Could you check a few things on this drawing? It's one solid part, dimensions in mm from its lowest x, y, z. A direction names the side the tool comes from. Give positions to 0.01 mm unless a question says otherwise; leave off trailing zeros. Order: outer loops, then holes, each group sorted by start corner. A loop starts at its lowest first (then second) coordinate and runs counter-clockwise, first axis right, second up. Notation, with made-up numbers: (40.5, -19.75) -> (92.5, -19.75) arc R7 ccw to (92.5, -10.75) -> close; hole circle Ø4 at (-27, -18). An arc over 180 degrees is marked (long way). Answer as a JSON object with one key per item and string values.
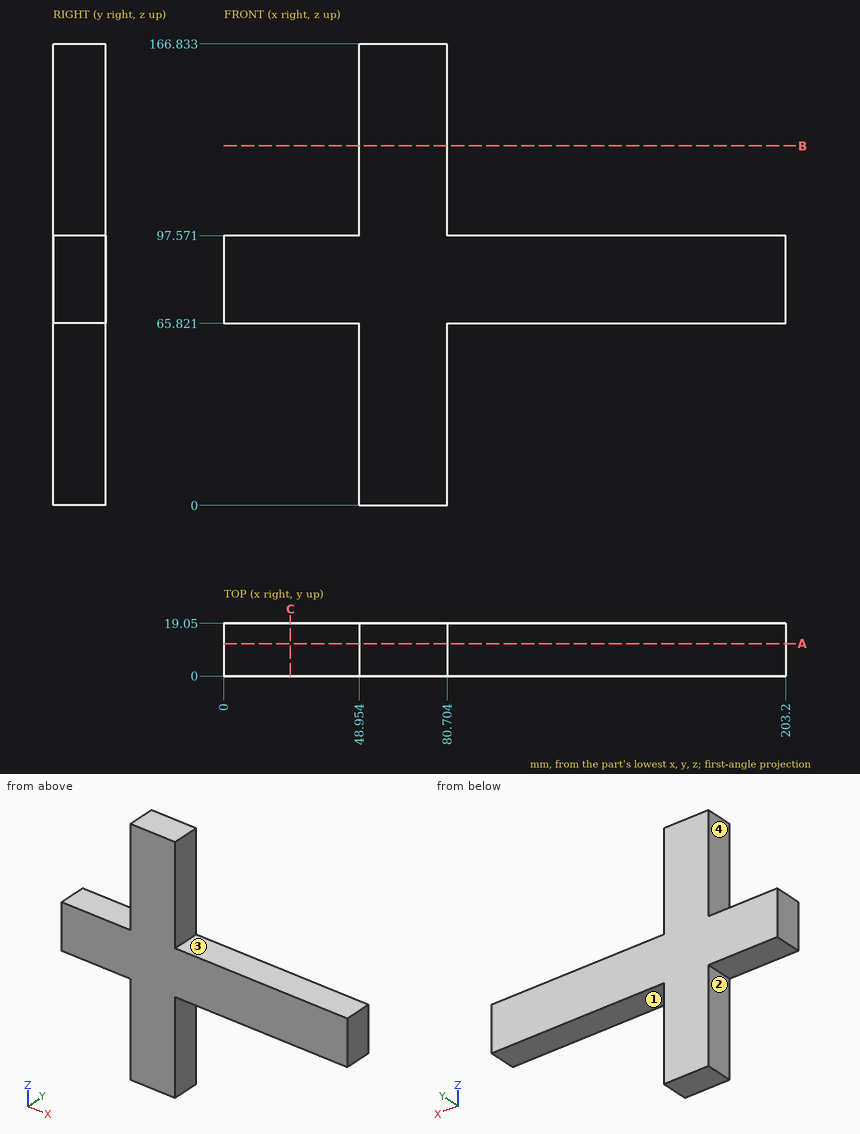
1. Please list where these lines run through material, in increasing order: L1, parallel to Z at x = 43, y = 10.25; L2, parallel to X at y = 15.75, z = 132.5.
Worked answers:
{"L1": "65.82 to 97.57", "L2": "48.95 to 80.7"}
2. If we section it at C-C on x = 24: Please give me the cut outline in (y, z).
Worked answers:
{"outline": "(0, 65.82) -> (19.05, 65.82) -> (19.05, 97.57) -> (0, 97.57) -> close"}
3. For the marked faces 1, 2, 3 and 4, which set-ups out of +Z, -Z, +X, -X, +Y, -Y let a thin tool reach every point of the face, with its end or its side?
Worked answers:
{"face 1": "-Z, +X, +Y, -Y", "face 2": "-Z, -X, +Y, -Y", "face 3": "+Z, +X, +Y, -Y", "face 4": "+Z, -X, +Y, -Y"}
4. Will these pins go through, and if not, where does the flat tip stop? pin 1 Ø1 at (y, z) = (13, 53.5) entering from +X; pin 2 Ø3 at (x, y) = (127.5, 15) entering from -Z; pin 3 Ø1 at (x, y) = (132, 13) entering from +Z; pin 4 Ø12 at (x, z) = (128.5, 108) entering from +Y.
Worked answers:
{"pin 1": "x = 80.7", "pin 2": "z = 65.82", "pin 3": "z = 97.57", "pin 4": "through"}
5. If we section it at B-B on z = 130: Please give me the cut outline in (x, y), then the cut area to 3 significant figures.
Worked answers:
{"outline": "(48.95, 0) -> (80.7, 0) -> (80.7, 19.05) -> (48.95, 19.05) -> close", "area": "605 mm²"}
6. If we section it at A-A on y = 11.75: Please give me the cut outline in (x, z).
Worked answers:
{"outline": "(0, 65.82) -> (48.95, 65.82) -> (48.95, 0) -> (80.7, 0) -> (80.7, 65.82) -> (203.2, 65.82) -> (203.2, 97.57) -> (80.7, 97.57) -> (80.7, 166.83) -> (48.95, 166.83) -> (48.95, 97.57) -> (0, 97.57) -> close"}
